from build123d import *

# Parameters (mm, degrees)
CROQUIS1_W              = 70
CROQUIS1_H              = 45
SALIENTE_EXTRUIR1_DEPTH = 5
REDONDEO1_R             = 10
REDONDEO2_R             = 10
CROQUIS2_R              = 17.5
SALIENTE_EXTRUIR2_DEPTH = 22
REDONDEO3_R             = 5
CROQUIS3_R              = 12.5
CORTAR_EXTRUIR1_DEPTH   = 50.60090725
CHAFL_N1_SIZE2          = 2.886751346
CHAFL_N1_SIZE           = 5
CROQUIS4_R              = 14.6
CORTAR_EXTRUIR2_DEPTH   = 2
CROQUIS5_R              = 4
CORTAR_EXTRUIR3_DEPTH   = 48.066442398


with BuildPart() as part:
    # Croquis1 → Saliente-Extruir1 (new body)
    with BuildSketch(Plane(origin=(0, 0, 0), x_dir=(1, 0, 0), z_dir=(0, 1, 0))):
        Rectangle(CROQUIS1_W, CROQUIS1_H)
    extrude(amount=SALIENTE_EXTRUIR1_DEPTH)

    # Redondeo1
    redondeo1_edges = [part.edges().sort_by_distance(p)[0] for p in [
        (35, 2.5, 22.5),
    ]]
    fillet(redondeo1_edges, radius=REDONDEO1_R)

    # Redondeo2
    redondeo2_edges = [part.edges().sort_by_distance(p)[0] for p in [
        (-35, 2.5, 22.5),
        (-35, 2.5, -22.5),
        (35, 2.5, -22.5),
    ]]
    fillet(redondeo2_edges, radius=REDONDEO2_R)

    # Croquis2 → Saliente-Extruir2 (add)
    with BuildSketch(Plane(origin=(0, 5, 0), x_dir=(1, 0, 0), z_dir=(0, 1, 0))):
        with Locations(Location((0, 0, 0), (0, 0, 270))):
            Circle(CROQUIS2_R)
    extrude(amount=SALIENTE_EXTRUIR2_DEPTH)

    # Redondeo3
    redondeo3_edges = [part.edges().sort_by_distance(p)[0] for p in [
        (0, 5, -17.5),
    ]]
    fillet(redondeo3_edges, radius=REDONDEO3_R - 0.0001)  # a hair under: the kernel refuses the full size

    # Croquis3 → Cortar-Extruir1 (cut, through all)
    with BuildSketch(Plane(origin=(0, 27, 0), x_dir=(1, 0, 0), z_dir=(0, 1, 0))):
        with Locations(Location((0, 0, 0), (0, 0, 270))):
            Circle(CROQUIS3_R)
    extrude(amount=-CORTAR_EXTRUIR1_DEPTH, mode=Mode.SUBTRACT)

    # Chaflán1
    chafl_n1_edges = [part.edges().sort_by_distance(p)[0] for p in [
        (0, 27, -12.5),
    ]]
    chafl_n1_side = [part.faces().sort_by_distance(p)[0] for p in [
        (0, 27, -12.557735027),
    ]]
    chamfer(chafl_n1_edges, length=CHAFL_N1_SIZE - 0.0001, length2=CHAFL_N1_SIZE2 - 0.0001, reference=chafl_n1_side[0])  # a hair under: the kernel refuses the full size

    # Croquis4 → Cortar-Extruir2 (cut)
    with BuildSketch(Plane(origin=(0, 0, 0), x_dir=(-1, 0, 0), z_dir=(0, -1, 0))):
        with Locations(Location((0, 0, 0), (0, 0, 90))):
            Circle(CROQUIS4_R)
    extrude(amount=-CORTAR_EXTRUIR2_DEPTH, mode=Mode.SUBTRACT)

    # Croquis5 → Cortar-Extruir3 (cut, through all)
    with BuildSketch(Plane(origin=(0, 5, 0), x_dir=(1, 0, 0), z_dir=(0, 1, 0))):
        with Locations(Location((-27.5, 0, 0), (0, 0, 270))):
            Circle(CROQUIS5_R)
        with Locations(Location((27.5, 0, 0), (0, 0, 270))):
            Circle(CROQUIS5_R)
    extrude(amount=-CORTAR_EXTRUIR3_DEPTH, mode=Mode.SUBTRACT)


solid = part.part
Geometry check sheet. Reference: the model listing, model coordinates, mm. A direction names the side the tool comes from. Coordinates: 2 decimals unless noted, no trailing zeros. Order: outer loops, then holes, each group sorted by start corner. A loop starts at its lowest first (then second) coordinate and runs counter-clockwise, first axis right, second up. Notation, with made-up numbers: (39.5, 30.5) - (53.5, 30.5) arc R20 cw to (53.5, 68.5) - close; hole circle Ø10 at (16, -28.75). An arc over 180 degrees is marked (long way). One line per item, written item: value.
(1) Sectioned sample at A-A (z = 0). Count the separate pieces of the cut face and the enclosed holes in it, and give its area (3 significant figures).
Data:
separate pieces: 4
enclosed holes: 0
area: 353 mm^2
(2) Release check for a two-part mould opening along X. For faces 1 (the face through (3.83, 24.25, 12.15)), 2 (the face through (31.99, 2.54, 19.65)), 3 (the face through (-32.15, 2.54, -19.49)) record: +X half, -X half, draft (parallel to the pull), parting line (faces both ways), or undercut.
Data:
face 1: undercut
face 2: +X half
face 3: -X half
(3) Depth check by flat-ended pin: pin 1 Ø5 at (x, z) = (-1, 11.5) entering from +Y; pin 2 Ø1.5 at (y, z) = (17, -7) entering from +X; pin 3 Ø20 at (x, z) = (0, 0) entering from -Y; pin 4 Ø6 at (x, z) = (6, 8) entering from +Y. Enter the tip coordinate at first touch or a pass-through.
Data:
pin 1: stops at y = 25
pin 2: stops at x = 16.35
pin 3: passes through
pin 4: stops at y = 24.4
(4) Sectioned sample at C-C (y = 11.5). Enter the section's corners in (x, z).
Data:
outline: circle Ø35 at (0, 0); hole circle Ø25 at (0, 0)
(5) Sectioned sample at D-D (x = -27.5). Enter the section's corners in (y, z), and give its area (3 significant figures).
Data:
outline: (0, -22.18) - (5, -22.18) - (5, -4) - (0, -4) - close; (0, 4) - (5, 4) - (5, 22.18) - (0, 22.18) - close
area: 182 mm^2
(6) Access from +Z, -Z, +X, -X, +Y, -Y to the whole of each face (thin tool, end or side, straight path). Record for faces 4 (the face through (7, 2, -11)), 5 (the face through (0, 2, -22.5)), 6 (the face through (-10.648, 18.381, -13.887)).
Data:
face 4: -Y
face 5: -Z, +X, -X, +Y, -Y
face 6: +Y
(7) Thickness scan on probe 1 along X at (y, z) = (1.5, 0); probe 2 along X at (y, z) = (2.75, 0); probe 3 along Y at (x, z) = (-20.5, 18). Record the ranges inside material, lowest first. Write a range as from..to.
Data:
probe 1: x = -35..-31.5, -23.5..-14.6, 14.6..23.5, 31.5..35
probe 2: x = -35..-31.5, -23.5..-12.5, 12.5..23.5, 31.5..35
probe 3: y = 0..5
